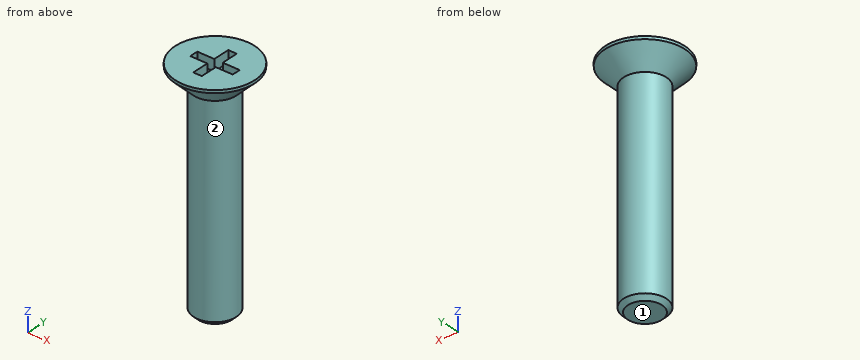
from build123d import *

# Parameters (mm, degrees)
SCHNITT_LINEAR_AUSTRAGEN1_DEPTH = 0.8
FASE1_SIZE                      = 0.3


with BuildPart() as part:
    # Skizze1 → Rotation1 (revolve)
    with BuildSketch(Plane(origin=(0, 0, 0), x_dir=(0, 0, -1), z_dir=(1, 0, 0))):
        Polygon((0, 0), (0, 2.8), (0.2, 2.8), (1.5, 1.5), (16, 1.5), (16, 0), align=None)
    revolve(axis=Axis((0, 0, 31.763581507), (0, 0, -1)))

    # Skizze3 → Schnitt-Linear austragen1 (cut)
    with BuildSketch(Plane.XY):
        Polygon((-1.5, -0.3), (-1.5, 0.3), (-0.3, 0.3), (-0.3, 1.5), (0.3, 1.5), (0.3, 0.3), (1.5, 0.3), (1.5, -0.3), (0.3, -0.3), (0.3, -1.5), (-0.3, -1.5), (-0.3, -0.3), align=None)
    extrude(amount=-SCHNITT_LINEAR_AUSTRAGEN1_DEPTH, mode=Mode.SUBTRACT)

    # Fase1
    fase1_edges = [part.edges().sort_by_distance(p)[0] for p in [
        (0, -1.5, -16),
    ]]
    chamfer(fase1_edges, length=FASE1_SIZE)


solid = part.part
Build history of the part. All positions in model axes, mm. Face numbers are marked on the shaded views. A direction names the side the tool comes from. Give positions to 0.01 mm unless a question says otherwise; leave off trailing zeros. Loops run counter-clockwise (first coordinate to the right, second up) from the corner with the lowest first, then second, coordinate; pieces in that order, holes last. Notation, with made-up numbers: (11, 41) -> (70, 41) arc R9 ccw to (70, 52) -> close; hole circle Ø6 at (31.5, 15). An arc over 180 degrees is marked (long way). Answer in a Markdown table with one row per item.
Item 1: Probe line 1 along Z through (x, y) = (0, 1.05); line 2 along Y through (x, z) = (-0.75, -9.5); line 3 along X through (y, z) = (-0.55, -8.75). List the from-to ranges inside material, lowest first. Write a range as [from, to].
Findings below:
| item | result |
|---|---|
| line 1 | z = [-16, -0.8] |
| line 2 | y = [-1.3, 1.3] |
| line 3 | x = [-1.4, 1.4] |
Item 2: Flat gauge pins, fed straight in: P1, Ø0.6, axis at y = -1, z = -0.5, coming from the +X side; P2, Ø1.5, axis at y = 0, z = -4, coming from the +X side; P3, Ø0.9, axis at x = 1, z = 0, coming from the -Y side. Where does each tip first touch, or does it go through?
Findings below:
| item | result |
|---|---|
| P1 | stops at x = 2.63 |
| P2 | stops at x = 1.5 |
| P3 | stops at y = -2.75 |
Item 3: Slice it at A-A on x = 0. Write the cut outline in (y, z), plus the area to 3 significant figures.
Findings below:
| item | result |
|---|---|
| outline | (-2.8, -0.2) -> (-1.5, -1.5) -> (-1.5, -15.7) -> (-1.2, -16) -> (1.2, -16) -> (1.5, -15.7) -> (1.5, -1.5) -> (2.8, -0.2) -> (2.8, 0) -> (1.5, 0) -> (1.5, -0.8) -> (-1.5, -0.8) -> (-1.5, 0) -> (-2.8, 0) -> close |
| area | 47.7 mm² |
Item 4: Tool access for the marked faces 1 and 2: list every direction of +Z, -Z, +X, -X, +Y, -Y with a clear straight run to the whole face (end or side of a thin tool).
Findings below:
| item | result |
|---|---|
| face 1 | -Z, +X, -X, +Y, -Y |
| face 2 | -Z |
Item 5: Slice it at C-C on z = -4.25. Write the cut outline in (x, y).
Findings below:
| item | result |
|---|---|
| outline | circle Ø3 at (0, 0) |
